Build history of the part. All positions in model axes, mm. Face numbers are marked on the shaded views. A direction names the side the tool comes from. Round coordinates to 2 decimals unless told otherwise and drop trailing zeros. Order: outer loops, then holes, each group sorted by start corner. A loop starts at its lowest first (then second) coordinate and runs counter-clockwise, first axis right, second up. Notation, with made-up numbers: (30.5, -28.5) -> (65.5, -28.5) arc R31 cw to (65.5, 10.5) -> close; hole circle Ø9 at (-31, 25). An arc over 180 degrees is marked (long way). Use a Markdown table: item, result. Add a question column.
Item 1: Slice it at D-D, the plane x = 6.75. Give the cut face in (y, z) (3 decimals).
Item 2: Pin check, flat tips, straight feed: pin 1 (12 mm diameter, centred on y = 9.5, z = -2.5, fed in from +X); pin 2 (6.5 mm diameter, centred on x = 2.5, z = 2.5, fed in from +Y); pin 3 (1.5 mm diameter, centred on x = 5, z = 8.5, fed in from -Y) (3 decimals); pin 4 (5 mm diameter, centred on x = 4, y = 15, fed in from +Z). Stop position of each tip, or through.
Item 3: 3-axis set-ups, long thin cutter, end or side, ignore diameter. For the marked faces 1, 2 and 3: which of +Z, -Z, +X, -X, +Y, -Y reach the whole face in a straight line?
Item 4: Slice it at C-C, the plane y = 8.5. Give the cut face in (x, z), plus the area to 3 significant figures.
Item 5: Probe L1, parallel to Y at x = -7.25, z = 5.5 (3 decimals); L2, parallel to X at y = 7.5, z = 0.25; L3, parallel to Y at x = -0.25, z = 2. List the from-to ranges inside material, lowest first.
Item 6: Two-plate mould, pull along X, no slides. Class the marked faces 4, 5 and 6: released by +X, released by -X, zero draft, split by the parting line, or undercut.
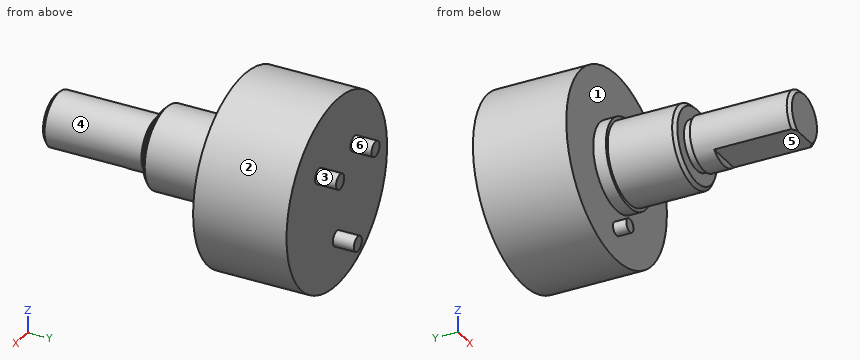
Autodesk Inventor part; units mm, degrees
ref_plane "YZ Plane" through (0, 0, 0) normal (1, 0, 0) x (0, 1, 0)
ref_plane "XZ Plane" through (0, 0, 0) normal (0, 1, 0) x (-1, 0, 0)
ref_plane "XY Plane" through (0, 0, 0) normal (0, 0, 1) x (1, 0, 0)
sketch "Sketch1" plane through (0, 0, 0) normal (0, 0, 1) x (1, 0, 0)
  line L0 (0, 0) -> (3.1712, 0)
  line L1 (3.1712, 0) -> (3.1712, 11.8618)
  line L2 (3.1712, 11.8618) -> (0, 11.8618)
  line L3 (0, 11.8618) -> (0, 0)
  line L4 (0, 11.8618) -> (2.9028, 11.8618)
  line L5 (2.9028, 11.8618) -> (2.9028, 12.7)
  line L6 (2.9028, 12.7) -> (0, 12.7)
  line L7 (0, 12.7) -> (0, 11.8618)
  line L8 (0, 12.7) -> (4.7625, 12.7)
  line L9 (4.7625, 12.7) -> (4.7625, 20.7264)
  line L10 (4.7625, 20.7264) -> (0, 20.7264)
  line L11 (0, 20.7264) -> (0, 12.7)
  line L12 (0, 20.7264) -> (5.1562, 20.7264)
  line L13 (5.1562, 20.7264) -> (5.1562, 22.225)
  line L14 (5.1562, 22.225) -> (0, 22.225)
  line L15 (0, 22.225) -> (0, 20.7264)
  line L16 (0, 22.225) -> (11.1125, 22.225)
  line L17 (11.1125, 22.225) -> (11.1125, 33.274)
  line L18 (11.1125, 33.274) -> (0, 33.274)
  line L19 (0, 33.274) -> (0, 22.225)
  dimension "d0" = 22.225
  dimension "d1" = 9.525
  dimension "d2" = 1.4986
  dimension "d3" = 0.8382
  dimension "d4" = 3.1712
  dimension "d5" = 5.1562
  dimension "d6" = 11.049
  dimension "d7" = 11.1125
  dimension "d8" = 4.7625
revolve "Revolution1" add sketch "Sketch1" angle 360 about axis through (0, 33.274, 0) along (0, -1, 0)
chamfer "Chamfer1" distance 0.3969 angle 45 2 edges at (-3.1712, 0, 0) (-4.7625, 12.7, 0)
sketch "Sketch2" plane through (0, 22.225, 0) normal (0, -1, 0) x (1, 0, 0)
  circle A0 centre (0, -7.366) radius 0.7874
  circle A1 centre (0, 0) radius 11.1125
  point P0 (0, 0)
  dimension "d13" = 1.5748
  dimension "d14" = 7.366
extrude "Extrusion1" add sketch "Sketch2" along normal blind 1.5748 contours A0
sketch "Sketch3" plane through (0, 0, 0) normal (0, -1, 0) x (1, 0, 0)
  line L0 (-2.1671, -2.3152) -> (2.1671, -2.3152)
  circle A0 centre (0, 0) radius 3.1712
  point P0 (0, 0)
  dimension "d18" = 5.4864
extrude "Extrusion2" cut sketch "Sketch3" against normal blind 9.525 contours L0 A0 picked at (-0.5411, -2.4515)
sketch "Sketch4" plane through (0, 33.274, 0) normal (0, 1, 0) x (1, 0, 0)
  circle A0 centre (0, 0) radius 5.5245 construction
  circle A1 centre (3.9116, -3.9012) radius 0.889
  circle A2 centre (-3.9116, -3.9012) radius 0.889
  circle A3 centre (0, 5.5245) radius 0.889
  line L0 (3.9116, -3.9012) -> (-3.9116, -3.9012) construction
  line L1 (0, 0) -> (0, 11.1125) construction
  circle A4 centre (0, 0) radius 11.1125 construction
  dimension "d21" = 11.049
  dimension "d22" = 7.8232
  dimension "d23" = 1.778
extrude "Extrusion3" add sketch "Sketch4" along normal blind 2.4892
properties part number "TT_Electronics_Encoder_6127V1A360L.5FS" material "Aluminum 6061"
Check sheet entries:
| question | item | result |
|---|---|---|
| 1 | outline | (22.225, -8.828) -> (33.274, -8.828) -> (33.274, 8.828) -> (22.225, 8.828) -> close |
| 2 | pin 1 | x = 4.76 |
| 2 | pin 2 | y = 35.76 |
| 2 | pin 3 | y = 22.225 |
| 2 | pin 4 | z = 4.52 |
| 3 | face 1 | -Y |
| 3 | face 2 | +Y, -Y |
| 3 | face 3 | +Y |
| 4 | outline | (-2.17, -2.32) -> (2.17, -2.32) arc R3.17 ccw (long way) to start |
| 4 | area | 29.0 mm2 |
| 5 | L1 | 22.225 to 33.274 |
| 5 | L2 | -3.16 to 3.16 |
| 5 | L3 | 0 to 33.27 |
| 6 | face 4 | split by the parting line |
| 6 | face 5 | zero draft |
| 6 | face 6 | undercut |
